The model under review builds one solid part; all positions refer to its coordinate system, in mm. A direction names the side the tool comes from. Coordinates: 2 decimals unless noted, no trailing zeros. Order: outer loops, then holes, each group sorted by start corner. A loop starts at its lowest first (then second) coordinate and runs counter-clockwise, first axis right, second up. Notation, with made-up numbers: M 45,78 L 64,78 A24 ccw 64,101 Z; hole C 10,62.25 d5. An arc over 180 degrees is marked long. Answer as CSV lines item,"result". Start each with the question number.
Q1. Machinability: for faces 1 (the face through (0.04, -30.52, 29.95)), 2 (the face through (2.5, -4, 39)), which of the approach directions +Z, -Z, +X, -X, +Y, -Y give a long, thin tool a straight path to every point of the face, cutting with its end or side? Answer none if there is none.
Q2. Consider section A-A on z = 0. Write out the cut boundary in (x, y) (1 decimal), and give its area (3 significant figures).
Q3. The part is to be moulded in two halves that separate along Y. For faces 3 (the face through (-2.5, -4, 39)), 4 (the face through (0, 40, -4.762)), 5 (the face through (0.04, 33.24, 0.1)), 6 (the face through (0.035, 48.453, -30.892)), say which applies: +Y half, -Y half, draft (parallel to the pull), parting line (faces both ways), or undercut.
Q4. Consider section D-D on z = 46. Write out the cut boundary in (x, y), and give its area (3 significant figures).
Q5. Consider section C-C on x = 0.2. State how many separate pieces and enclosed holes the cut face has, and give its area (3 significant figures).
Q6. For P1, Ø3, axis at x = 0, y = -27, coming from the -Z side; P2, Ø2, axis at x = 1, z = -40, coming from the +Y side; P3, Ø2, axis at x = -0.5, y = -39, coming from the +Z side; P4, Ø1.5, axis at y = 30.5, z = 26.5, coming from the -X side, all flat-tipped, find the tip position at first contact; note any pin that passes through.
Q7. Wall thickness on L1, parallel to Y at x = -1.15, z = 0 (1 decimal); L2, parallel to Y at x = -1.1, z = 38 (1 decimal); L3, parallel to Y at x = -1.75, z = -34: over which ranges is each line inside the solid? List them lowest first. Write a range as [from, to].
Q8. Consider section B-B on z = -18. Write out the cut boundary in (x, y).
from build123d import *

# Parameters (mm, degrees)
SKETCH1_R           = 57.463033318
SKETCH1_R_2         = 42.7625
SKETCH1_R_3         = 3.175
BOSS_EXTRUDE1_DEPTH = 2.5


with BuildPart() as part:
    # Sketch1 → Boss-Extrude1 (new body, symmetric)
    with BuildSketch(Plane(origin=(0, 0, 0), x_dir=(0, 0, -1), z_dir=(1, 0, 0))):
        Circle(SKETCH1_R)
        Circle(SKETCH1_R_2, mode=Mode.SUBTRACT)
        with BuildLine():
            Line((-38, 4.7625), (-42.496470442, 4.7625))
            ThreePointArc((-42.496470442, 4.7625), (-42.7625, 0), (-42.496470442, -4.7625))
            Line((-42.496470442, -4.7625), (-38, -4.7625))
            ThreePointArc((-38, -4.7625), (-33.2375, 0), (-38, 4.7625))
        make_face()
        with Locations((-38, 0)):
            Circle(SKETCH1_R_3, mode=Mode.SUBTRACT)
        with BuildLine():
            ThreePointArc((4.7625, 42.496470442), (0, 42.7625), (-4.7625, 42.496470442))
            Line((-4.7625, 42.496470442), (-4.7625, 38))
            ThreePointArc((-4.7625, 38), (0, 33.2375), (4.7625, 38))
            Line((4.7625, 38), (4.7625, 42.496470442))
        make_face()
        with Locations((0, 38)):
            Circle(SKETCH1_R_3, mode=Mode.SUBTRACT)
        with BuildLine():
            ThreePointArc((42.7625, 0), (42.695940811, 2.384962158), (42.496470442, 4.7625))
            Line((42.496470442, 4.7625), (38, 4.7625))
            ThreePointArc((38, 4.7625), (33.2375, 0), (38, -4.7625))
            Line((38, -4.7625), (42.496470442, -4.7625))
            ThreePointArc((42.496470442, -4.7625), (42.695940811, -2.384962158), (42.7625, 0))
        make_face()
        with Locations((38, 0)):
            Circle(SKETCH1_R_3, mode=Mode.SUBTRACT)
        with BuildLine():
            Line((-4.7625, -38), (-4.7625, -42.496470442))
            ThreePointArc((-4.7625, -42.496470442), (0, -42.7625), (4.7625, -42.496470442))
            Line((4.7625, -42.496470442), (4.7625, -38))
            ThreePointArc((4.7625, -38), (0, -33.2375), (-4.7625, -38))
        make_face()
        with Locations((0, -38)):
            Circle(SKETCH1_R_3, mode=Mode.SUBTRACT)
    extrude(amount=BOSS_EXTRUDE1_DEPTH, both=True)


solid = part.part
Evaluation:
1,face 1,"+X, -X"
1,face 2,"+Z, -Z, +X, +Y, -Y"
2,outline,"M -2.5,-57.5 L 2.5,-57.5 L 2.5,-41.2 L -2.5,-41.2 Z; M -2.5,-34.8 L 2.5,-34.8 L 2.5,-33.2 L -2.5,-33.2 Z; M -2.5,33.2 L 2.5,33.2 L 2.5,34.8 L -2.5,34.8 Z; M -2.5,41.2 L 2.5,41.2 L 2.5,57.5 L -2.5,57.5 Z"
2,area,"179 mm²"
3,face 3,"draft"
3,face 4,"undercut"
3,face 5,"undercut"
3,face 6,"parting line"
4,outline,"M -2.5,-34.44 L 2.5,-34.44 L 2.5,34.44 L -2.5,34.44 Z"
4,area,"344 mm²"
5,separate pieces,"1"
5,enclosed holes,"5"
5,area,"4,820 mm²"
6,P1,"stops at z = -51.5"
6,P2,"stops at y = 42.2"
6,P3,"stops at z = 43.1"
6,P4,"passes through"
7,L1,"y = [-57.5, -41.2], [-34.8, -33.2], [33.2, 34.8], [41.2, 57.5]"
7,L2,"y = [-43.1, -19.6], [-4.8, -3.2], [3.2, 4.8], [19.6, 43.1]"
7,L3,"y = [-46.32, -25.94], [-2.58, 2.58], [25.94, 46.32]"
8,outline,"M -2.5,-54.57 L 2.5,-54.57 L 2.5,-38.79 L -2.5,-38.79 Z; M -2.5,38.79 L 2.5,38.79 L 2.5,54.57 L -2.5,54.57 Z"
